Solid Edge part; units mm, degrees
sketch "Sketch1" plane through (0, 0, 0) normal (0, 0, 1) x (1, 0, 0)
  circle A0 centre (247.2981, 19.0036) radius 1.75
  circle A1 centre (285.344, 19.0031) radius 1.75
  circle A2 centre (266.3208, -0.0196) radius 30.9975
  circle A3 centre (274.8439, 8.5032) radius 1.7
  circle A4 centre (257.798, 8.5035) radius 1.7
  circle A5 centre (257.7977, -8.5424) radius 1.7
  circle A6 centre (274.8436, -8.5427) radius 1.7
  circle A7 centre (285.3435, -19.0428) radius 1.7
  circle A8 centre (247.2976, -19.0423) radius 1.7
extrude "Protrusion1" add sketch "Sketch1" along normal blind 2.6
sketch "Sketch2" plane through (0, 0, 2.6) normal (0, 0, 1) x (1, 0, 0)
  circle A0 centre (257.798, 8.5035) radius 2.5
  circle A1 centre (274.8439, 8.5032) radius 2.5
  circle A2 centre (274.8436, -8.5427) radius 2.5
  circle A3 centre (257.7977, -8.5424) radius 2.5
extrude "Cutout1" cut sketch "Sketch2" against normal blind 2
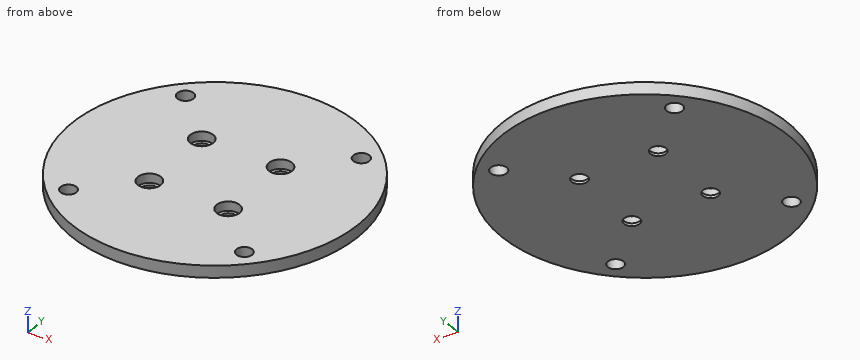
Input: part model. Units: mm. Frame: model coordinates. Give positions to 0.01 mm unless a question says otherwise; leave off trailing zeros. Write each loop counter-clockwise with the first axis right and the second up, starting at its lowest first coordinate (ties: lowest second). Pieces come first, ordered by that corner, then holes. Notation, with made-up numbers: M 27.25,26.5 L 57.25,26.5 A18 cw 57.25,59.5 Z; hole C -12.75,5 d4. An arc over 180 degrees is marked long. Write item = value, one per line. Start each with the question number.
1) First-contact query: pin 1 Ø1.5 at (x, y) = (256.5, 9) entering from +Z. Flat tip, straight axial feed; report the tip coordinate or a pass-through.
2) Cut plane A-A on z = 1.8. Count the separate pieces of the cut face and the enclosed holes in it, then the cut area to 3 significant figures.
3) Cut plane B-B on y = -23. Return the cut outline in (x, z), then the cut area to 3 significant figures.
4) Material intervals for line 1 along X through (y, z) = (-7, 0.1); line 2 along X through (y, z) = (-18, 2); line 3 along Y through (x, z) = (284, 0.75), sorted ascending. Write a range as [from, to].
5) Cut plane C-C on x = 280.5. Return the cut outline in (y, z), then the cut area to 3 significant figures.
Solved:
q1.pin_1 = 0.6
q2.separate_pieces = 1
q2.enclosed_holes = 8
q2.area = 2,900 mm2
q3.outline = M 245.52,0 L 287.12,0 L 287.12,2.6 L 245.52,2.6 Z
q3.area = 108 mm2
q4.line_1 = [236.12, 257.08], [258.51, 274.13], [275.56, 296.52]
q4.line_2 = [241.07, 245.95], [248.64, 284], [286.69, 291.57]
q4.line_3 = [-25.48, -20.08], [-18, 17.88], [20.12, 25.44]
q5.outline = M -27.58,0 L 27.54,0 L 27.54,2.6 L -27.58,2.6 Z
q5.area = 143 mm2
